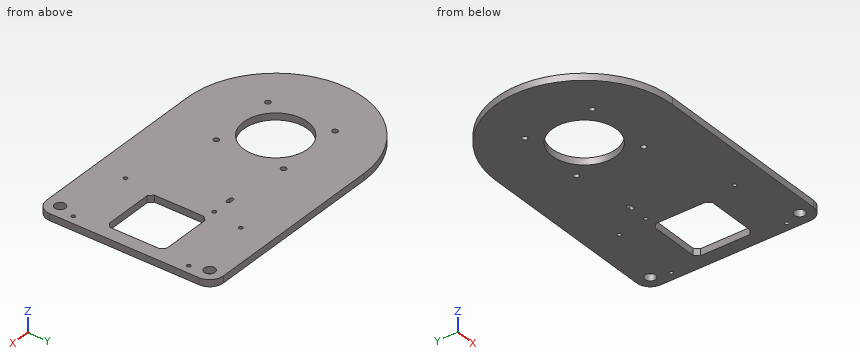
from build123d import *

# Parameters (mm, degrees)
SKETCH1_R           = 3.9
SKETCH1_R_2         = 23.48
SKETCH1_R_3         = 1.975
SKETCH1_R_4         = 1.4
BOSS_EXTRUDE4_DEPTH = 5


with BuildPart() as part:
    # Sketch1 → Boss-Extrude4 (new body)
    with BuildSketch(Plane.XY):
        with BuildLine():
            Line((-40, -65), (95, -65))
            ThreePointArc((95, -65), (102.071067812, -62.071067812), (105, -55))
            Line((105, -55), (105, 55))
            ThreePointArc((105, 55), (102.071067812, 62.071067812), (95, 65))
            Line((95, 65), (-40, 65))
            ThreePointArc((-40, 65), (-105, 0), (-40, -65))
        make_face()
        with Locations((95, 55)):
            Circle(SKETCH1_R, mode=Mode.SUBTRACT)
        with Locations((95, -55)):
            Circle(SKETCH1_R, mode=Mode.SUBTRACT)
        with Locations((-40, 0)):
            Circle(SKETCH1_R_2, mode=Mode.SUBTRACT)
        with Locations((-64.75, 24.75)):
            Circle(SKETCH1_R_3, mode=Mode.SUBTRACT)
        with Locations((-15.25, 24.75)):
            Circle(SKETCH1_R_3, mode=Mode.SUBTRACT)
        with Locations((-15.25, -24.75)):
            Circle(SKETCH1_R_3, mode=Mode.SUBTRACT)
        with Locations((-64.75, -24.75)):
            Circle(SKETCH1_R_3, mode=Mode.SUBTRACT)
        with Locations((98.75, 42.5)):
            Circle(SKETCH1_R_4, mode=Mode.SUBTRACT)
        with Locations((48.75, 42.5)):
            Circle(SKETCH1_R_4, mode=Mode.SUBTRACT)
        with Locations((48.75, -42.5)):
            Circle(SKETCH1_R_4, mode=Mode.SUBTRACT)
        with Locations((98.75, -42.5)):
            Circle(SKETCH1_R_4, mode=Mode.SUBTRACT)
        with Locations((45, 20)):
            Circle(SKETCH1_R_4, mode=Mode.SUBTRACT)
        Polygon((95, 18.25), (95, -18.25), (92, -21.25), (55.5, -21.25), (52.5, -18.25), (52.5, 18.25), (55.5, 21.25), (92, 21.25), align=None, mode=Mode.SUBTRACT)
        with BuildLine():
            Line((28.6, 21.4), (31.4, 21.4))
            ThreePointArc((31.4, 21.4), (32.8, 20), (31.4, 18.6))
            Line((31.4, 18.6), (28.6, 18.6))
            ThreePointArc((28.6, 18.6), (27.2, 20), (28.6, 21.4))
        make_face(mode=Mode.SUBTRACT)
    extrude(amount=BOSS_EXTRUDE4_DEPTH)


solid = part.part
The listing builds one solid part. Answer for the finished solid, in the listing's coordinates (mm). Give positions to 0.01 mm unless a question says otherwise; leave off trailing zeros. Order: outer loops, then holes, each group sorted by start corner. A loop starts at its lowest first (then second) coordinate and runs counter-clockwise, first axis right, second up. Notation, with made-up numbers: (-31.75, 53) -> (-3.75, 53) arc R13 ccw to (-3.75, 66) -> close; hole circle Ø2 at (56.5, 81.25). An arc over 180 degrees is marked (long way). Put each result on its own line as item: value.
Item 1: A cutting plane is placed at C-C on x = -32. Give the vertices of the cut face in (y, z), plus the area to 3 significant figures.
Established:
outline: (-65, 0) -> (-22.08, 0) -> (-22.08, 5) -> (-65, 5) -> close; (22.08, 0) -> (65, 0) -> (65, 5) -> (22.08, 5) -> close
area: 429 mm^2
Item 2: A cutting plane is placed at B-B on z = 3.95. Count the separate pieces of the cut face and the enclosed holes in it, plus the area to 3 significant figures.
Established:
separate pieces: 1
enclosed holes: 14
area: 21,700 mm^2
Item 3: Given P1, Ø4.5, axis at x = 95, y = -55, coming from the -Z side, flat-ended and moving along its own axis, determine where the tip first touches the part or whether it passes through.
Established:
P1: passes through
Item 4: A cutting plane is placed at A-A on y = 0. Give the vertices of the cut face in (x, z), plus the area to 3 significant figures.
Established:
outline: (-105, 0) -> (-63.48, 0) -> (-63.48, 5) -> (-105, 5) -> close; (-16.52, 0) -> (52.5, 0) -> (52.5, 5) -> (-16.52, 5) -> close; (95, 0) -> (105, 0) -> (105, 5) -> (95, 5) -> close
area: 603 mm^2
Item 5: Straight lines are drawn through the part: line 1 (X direction, y = -1.5, z = 1.25); line 2 (Y direction, x = 48.75, z = 2.4); line 3 (Y direction, x = -15.25, z = 1.6) (3 decimals). For each, find the intervals that lie inside material, in ascending order.
Established:
line 1: x = -104.98 to -63.43, -16.57 to 52.5, 95 to 105
line 2: y = -65 to -43.9, -41.1 to 41.1, 43.9 to 65
line 3: y = -65 to -26.725, -22.775 to 22.775, 26.725 to 65
